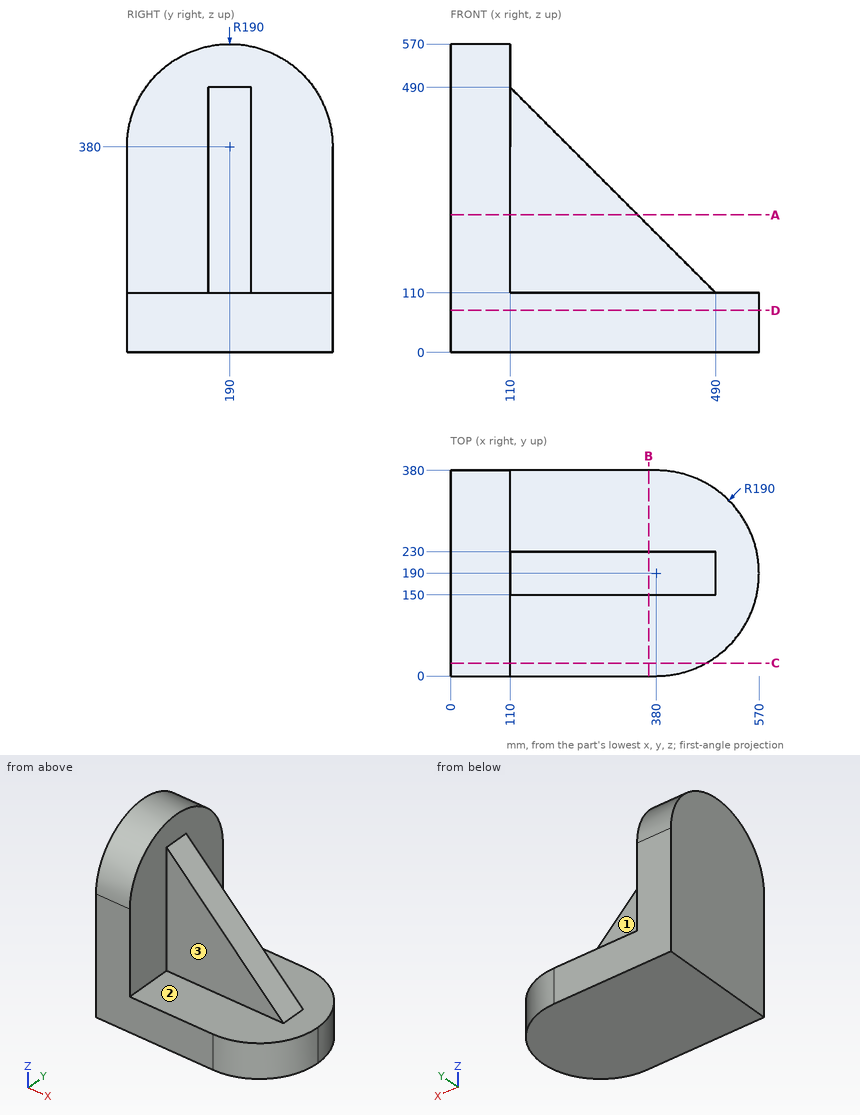
The figure shows three views and two pictorial views of one solid part (mm, origin at its lowest corner). Answer the questions. A direction names the side the tool comes from. Give positions to 0.01 mm unless a question says otherwise; leave off trailing zeros. Write each loop counter-clockwise with the first axis right and the second up, starting at its lowest first coordinate (ties: lowest second). Pieces come first, ordered by that corner, then holes. Notation, with made-up numbers: M 73,-11 L 107,-11 A25 cw 107,28 Z; hole C 82.25,30 d3. An arc over 180 degrees is marked long. Write each question's results on one line, items separated by ' | '.
Q1. Section B-B, the plane x = 366 is taken. Write down the section's boundary in (y, z), then the cut area to 3 significant figures.
Output values:
outline: M 0,0 L 380,0 L 380,110 L 230,110 L 230,234 L 150,234 L 150,110 L 0,110 Z | area: 51,700 mm2
Q2. Flat-ended cylindrical pins translate along their axes: P1, Ø6, axis at x = 282, y = 51, coming from the -Z side; P2, Ø12, axis at y = 141.5, z = 249.5, coming from the +X side; P3, Ø2, axis at x = 303, y = 61.5, coming from the +Z side; P4, Ø1, axis at x = 181.5, z = 387.5, coming from the +Y side. Find the tip coordinate at first contact, or state that the pin passes through.
Output values:
P1: z = 0 | P2: x = 110 | P3: z = 110 | P4: y = 230
Q3. Section A-A, the plane z = 254 is taken. Write down the section's boundary in (x, y).
Output values:
outline: M 0,0 L 110,0 L 110,150 L 346,150 L 346,230 L 110,230 L 110,380 L 0,380 Z
Q4. Section C-C, the plane y = 24 is taken. Write down the section's boundary in (x, z), then the cut area to 3 significant figures.
Output values:
outline: M 0,0 L 472.43,0 L 472.43,110 L 110,110 L 110,472.43 L 0,472.43 Z | area: 91,800 mm2
Q5. A tool of negligible diameter and unlimited length cuts with its end or side. For the marked faces 1, 2 and 3, from which of +Z, -Z, +X, -X, +Y, -Y can it reach the whole face along a straight path? Write none if from no direction.
Output values:
face 1: +Z, +X, +Y | face 2: +Z, +X | face 3: +Z, +X, -Y
Q6. Consider L1, parallel to Z at x = 430, y = 60; L2, parallel to Y at x = 379.5, z = 131. Determine where each line is inside the solid, lowest interval first. Write a range as from..to.
Output values:
L1: 0..110 | L2: 150..230
Q7. Section D-D, the plane z = 77.5 is taken. Write down the section's boundary in (x, y).
Output values:
outline: M 0,0 L 380,0 A190 ccw 380,380 L 0,380 Z
